```python
from build123d import *

# Parameters (mm, degrees)
F1_R     = 10.5
F2_DEPTH = 15
F3_R     = 13
F4_DEPTH = 2


# Not quite as in the source:
# - a fillet or chamfer that OpenCascade refuses, or shapes differently, is made with other operations: its cross-section is extruded or revolved along the edge and cut away or added


with BuildPart() as f2:
    # F1 (on face) → F2 (new body)
    with BuildSketch(Plane.YZ):
        Circle(F1_R)
    extrude(amount=F2_DEPTH)

    # F3 (on face) → F4 (join)
    with BuildSketch(Plane.YZ):
        Circle(F3_R)
    extrude(amount=-F4_DEPTH)

    # F5: fillet of radius 3 on 1 edges, made by hand

    # F5_s1 → F5_t2 (revolve, cut)
    with BuildSketch(Plane.XY):
        with BuildLine():
            ThreePointArc((0, 13), (-1.4494897428, 11.9036236828), (-2, 10.1715728753))
            Line((-2, 10.1715728753), (-2, 13))
            Line((-2, 13), (0, 13))
        make_face()
    revolve(axis=Axis((-2, 0, 0), (1, 0, 0)), mode=Mode.SUBTRACT)


solid = f2.part
```
Input: part model. Units: mm. Frame: model coordinates. A direction names the side the tool comes from. Give positions to 0.01 mm unless a question says otherwise; leave off trailing zeros. Order: outer loops, then holes, each group sorted by start corner. A loop starts at its lowest first (then second) coordinate and runs counter-clockwise, first axis right, second up. Notation, with made-up numbers: (59, 72.5) -> (116, 72.5) arc R27 ccw to (116, 107.5) -> close; hole circle Ø11 at (-9.5, -11). An arc over 180 degrees is marked (long way). Write each question's results on one line, items separated by ' | '. Start each with the question number.
Item 1: Cut plane A-A on y = 0. Return the cut outline in (x, z), then the cut area to 3 significant figures.
Item 2: Set-up query: faces 1 (the flat face through (0, -9, 6)), 2 (the flat face through (15, 0, 0)). Return all of +Z, -Z, +X, -X, +Y, -Y with unobstructed straight access to the full face (end or side cutting, diameter ignored); none if empty.
Item 3: Line query: line 1 (Y direction, x = 3.5, z = -3); line 2 (Y direction, x = 8.5, z = 5.25); line 3 (Z direction, x = 3.75, y = 2.75). Output: solid intervals per line, ascending.
Item 4: Cut plane C-C on x = 1. Return the cut outline in (y, z).
Item 5: Contact query for flat-ended pins moving along their axis: P1, Ø5, axis at x = 12.5, y = -4, coming from the +Z side; P2, Ø1, axis at x = 8.5, z = -5.5, coming from the -Y side; P3, Ø2, axis at x = 4.5, y = -1, coming from the +Z side. Output: stop coordinate, or through.
Established:
1) outline: (-2, -10.17) arc R3 ccw to (0, -13) -> (0, -10.5) -> (15, -10.5) -> (15, 10.5) -> (0, 10.5) -> (0, 13) arc R3 ccw to (-2, 10.17) -> close | area: 364 mm^2
2) face 1: +X | face 2: +Z, -Z, +X, +Y, -Y
3) line 1: -10.06 to 10.06 | line 2: -9.09 to 9.09 | line 3: -10.13 to 10.13
4) outline: circle Ø21 at (0, 0)
5) P1: z = 10.39 | P2: y = -9.23 | P3: z = 10.5
